from build123d import *

# Parameters (mm, degrees)
SKETCH1_W                 = 30
SKETCH1_H                 = 28
SKETCH1_R                 = 11
BOSS_EXTRUDE1_DEPTH       = 7
SKETCH2_W                 = 5
SKETCH2_H                 = 2.5
BOSS_EXTRUDE2_DEPTH       = 13
CHAMFER2_SIZE             = 2
BOSS_EXTRUDE6_DEPTH       = 2.5
CHAMFER3_SIZE             = 2
CHAMFER4_SIZE             = 2
BOSS_EXTRUDE4_DEPTH       = 2.5
CHAMFER6_SIZE             = 2.5
CHAMFER7_SIZE             = 7
CHAMFER7_SIZE_2           = 13.165085257
SKETCH7_R                 = 1.5
CUT_EXTRUDE2_DEPTH        = 6.4
BOSS_EXTRUDE7_START       = -2.5
SKETCH8_W                 = 30
SKETCH8_H                 = 5
BOSS_EXTRUDE7_DEPTH       = 4.5
CHAMFER8_SIZE             = 4.000836323
CHAMFER8_SIZE_2           = 2.5
CUT_EXTRUDE3_START        = -3
SKETCH9_R                 = 1.5
CUT_EXTRUDE3_DEPTH        = 3
SKETCH10_W                = 5.5
SKETCH10_H                = 3
CUT_EXTRUDE4_DEPTH        = 5.6
CUT_EXTRUDE5_START        = -30
SKETCH10_2_W              = 5.5
SKETCH10_2_H              = 3
CUT_EXTRUDE5_DEPTH        = 5.6
F_1_0MM_DOWEL_HOLE1_D     = 3
F_1_0MM_DOWEL_HOLE1_DEPTH = 7.098709071
F_1_0MM_DOWEL_HOLE1_TIP   = 0.901290929


with BuildPart() as part:
    # Sketch1 → Boss-Extrude1 (new body)
    with BuildSketch(Plane.XY):
        Rectangle(SKETCH1_W, SKETCH1_H)
        Circle(SKETCH1_R, mode=Mode.SUBTRACT)
    extrude(amount=BOSS_EXTRUDE1_DEPTH)

    # Sketch2 → Boss-Extrude2 (add)
    with BuildSketch(Plane(origin=(0, 0, 0), x_dir=(-1, 0, 0), z_dir=(0, 0, -1))):
        with Locations((-12.5, -12.75)):
            Rectangle(SKETCH2_W, SKETCH2_H)
        with Locations((12.5, -12.75)):
            Rectangle(SKETCH2_W, SKETCH2_H)
    extrude(amount=BOSS_EXTRUDE2_DEPTH)

    # Chamfer2
    chamfer2_edges = [part.edges().sort_by_distance(p)[0] for p in [
        (-10, -12.75, 0),
        (10, -12.75, 0),
    ]]
    chamfer(chamfer2_edges, length=CHAMFER2_SIZE)

    # Sketch5 → Boss-Extrude6 (add)
    with BuildSketch(Plane.XZ.offset(14)):
        Polygon((-10, -2), (-10, -7.5), (10, -7.5), (10, -2), (8, 0), (-8, 0), align=None)
    extrude(amount=-BOSS_EXTRUDE6_DEPTH)

    # Chamfer3
    chamfer3_edges = [part.edges().sort_by_distance(p)[0] for p in [
        (15, 0, 7),
    ]]
    chamfer(chamfer3_edges, length=CHAMFER3_SIZE)

    # Chamfer4
    chamfer4_edges = [part.edges().sort_by_distance(p)[0] for p in [
        (-15, 0, 7),
    ]]
    chamfer(chamfer4_edges, length=CHAMFER4_SIZE)

    # Sketch4 → Boss-Extrude4 (add)
    with BuildSketch(Plane(origin=(0, 0, 0), x_dir=(-1, 0, 0), z_dir=(0, 0, -1))):
        Polygon((-15, 0), (15, 11.5), (15, 14), (-15, 14), align=None)
    extrude(amount=BOSS_EXTRUDE4_DEPTH)

    # Chamfer6
    # the kernel refuses this chamfer: 2.5 mm, written as the material it adds along each edge
    with BuildSketch(Plane(origin=(21.003247512, -2.30124488, 0), x_dir=(-0.3578006820796162, -0.9333930836859554, 0.02749587661058638), z_dir=(-0.9337461173020497, 0.35793601163245237, 0))) as chamfer6_piece_1_section:
        Polygon((CHAMFER6_SIZE * 0.999621916911, -CHAMFER6_SIZE * 0.0274958766106), (-CHAMFER6_SIZE * 0.0274958766106, -CHAMFER6_SIZE * 0.999621916911), (0, 0), align=None)
    chamfer6_piece_1 = extrude(amount=17.263908412, mode=Mode.PRIVATE)
    chamfer6_piece_1 = chamfer6_piece_1 - Plane(origin=(0, 0, -0.835393566), x_dir=(1, 0, 0), z_dir=(0, 0, -1)) * Cylinder(11, 45, mode=Mode.PRIVATE)
    chamfer6_piece_1 = split(chamfer6_piece_1, bisect_by=Plane(origin=(15, -0.113968884, -0.835393566), z_dir=(-1, 0, 0)), keep=Keep.TOP, mode=Mode.PRIVATE)
    add(chamfer6_piece_1)
    with BuildSketch(Plane(origin=(-1.03959441, 6.148511191, 0), x_dir=(-0.35780068207961624, -0.9333930836859554, 0.02749587661058638), z_dir=(-0.9337461173020497, 0.35793601163245237, 0))) as chamfer6_piece_2_section:
        Polygon((CHAMFER6_SIZE * 0.999621916911, -CHAMFER6_SIZE * 0.0274958766106), (-CHAMFER6_SIZE * 0.0274958766106, -CHAMFER6_SIZE * 0.999621916911), (0, 0), align=None)
    chamfer6_piece_2 = extrude(amount=21.380172546, mode=Mode.PRIVATE)
    chamfer6_piece_2 = chamfer6_piece_2 - Plane(origin=(0, 0, -0.851534645), x_dir=(1, 0, 0), z_dir=(0, 0, -1)) * Cylinder(11, 53, mode=Mode.PRIVATE)
    chamfer6_piece_2 = split(chamfer6_piece_2, bisect_by=Plane(origin=(-15, 9.244820467, -0.851534645), z_dir=(1, 0, 0)), keep=Keep.TOP, mode=Mode.PRIVATE)
    add(chamfer6_piece_2)

    # Chamfer7
    # the kernel refuses this chamfer: 13.165085257, 7 mm, written as the material it adds along each edge
    with BuildSketch(Plane(origin=(-15, -11.5, 0), x_dir=(0, 0.9979482451756082, 0.06402577567608186), z_dir=(1, 0, 0))) as chamfer7_piece_1_section:
        Polygon((CHAMFER7_SIZE * 0.997948245176, -CHAMFER7_SIZE * 0.0640257756761), (-CHAMFER7_SIZE_2 * 0.0640257756781, -CHAMFER7_SIZE_2 * 0.997948245208), (0, 0), align=None)
    chamfer7_piece_1 = extrude(amount=30, mode=Mode.PRIVATE)
    chamfer7_piece_1 = chamfer7_piece_1 - Plane(origin=(0, 0, -3.073682767), x_dir=(1, 0, 0), z_dir=(0, 0, -1)) * Cylinder(11, 113, mode=Mode.PRIVATE)
    chamfer7_piece_1 = split(chamfer7_piece_1, bisect_by=Plane(origin=(-10, -8.887755394, -3.073682767), z_dir=(-1, 0, 0)), keep=Keep.TOP, mode=Mode.PRIVATE)
    chamfer7_piece_1 = split(chamfer7_piece_1, bisect_by=Plane(origin=(-12.500128058, -8.887755394, -7.5), z_dir=(0, 0, 1)), keep=Keep.TOP, mode=Mode.PRIVATE)
    add(chamfer7_piece_1)
    with BuildSketch(Plane(origin=(-15, -11.5, 0), x_dir=(0, 0.9979482451756082, 0.06402577567608186), z_dir=(1, 0, 0))) as chamfer7_piece_2_section:
        Polygon((CHAMFER7_SIZE * 0.997948245176, -CHAMFER7_SIZE * 0.0640257756761), (-CHAMFER7_SIZE_2 * 0.0640257756781, -CHAMFER7_SIZE_2 * 0.997948245208), (0, 0), align=None)
    chamfer7_piece_2 = extrude(amount=30, mode=Mode.PRIVATE)
    chamfer7_piece_2 = split(chamfer7_piece_2, bisect_by=Plane(origin=(-10, -10.721530873, -9.597564575), z_dir=(-1, 0, 0)), keep=Keep.TOP, mode=Mode.PRIVATE)
    chamfer7_piece_2 = split(chamfer7_piece_2, bisect_by=Plane(origin=(-12.5, -10.721530873, -7.5), z_dir=(0, 0, -1)), keep=Keep.TOP, mode=Mode.PRIVATE)
    chamfer7_piece_2 = split(chamfer7_piece_2, bisect_by=Plane(origin=(-12.5, -10.721530873, -13), z_dir=(0, 0, 1)), keep=Keep.TOP, mode=Mode.PRIVATE)
    add(chamfer7_piece_2)
    with BuildSketch(Plane(origin=(-15, -11.5, 0), x_dir=(0, 0.9979482451756082, 0.06402577567608186), z_dir=(1, 0, 0))) as chamfer7_piece_3_section:
        Polygon((CHAMFER7_SIZE * 0.997948245176, -CHAMFER7_SIZE * 0.0640257756761), (-CHAMFER7_SIZE_2 * 0.0640257756781, -CHAMFER7_SIZE_2 * 0.997948245208), (0, 0), align=None)
    chamfer7_piece_3 = extrude(amount=30, mode=Mode.PRIVATE)
    chamfer7_piece_3 = chamfer7_piece_3 - Plane(origin=(0, 0, -3.793876077), x_dir=(1, 0, 0), z_dir=(0, 0, -1)) * Cylinder(11, 113, mode=Mode.PRIVATE)
    chamfer7_piece_3 = split(chamfer7_piece_3, bisect_by=Plane(origin=(-10, -6.598719884, -3.793876077), z_dir=(1, 0, 0)), keep=Keep.TOP, mode=Mode.PRIVATE)
    chamfer7_piece_3 = split(chamfer7_piece_3, bisect_by=Plane(origin=(-9.499486782, -6.598719884, -7.5), z_dir=(0, 0, 1)), keep=Keep.TOP, mode=Mode.PRIVATE)
    chamfer7_piece_3 = split(chamfer7_piece_3, bisect_by=Plane(origin=(10, -6.598719884, -3.793876077), z_dir=(-1, 0, 0)), keep=Keep.TOP, mode=Mode.PRIVATE)
    add(chamfer7_piece_3)
    with BuildSketch(Plane(origin=(-15, -11.5, 0), x_dir=(0, 0.9979482451756082, 0.06402577567608186), z_dir=(1, 0, 0))) as chamfer7_piece_4_section:
        Polygon((CHAMFER7_SIZE * 0.997948245176, -CHAMFER7_SIZE * 0.0640257756761), (-CHAMFER7_SIZE_2 * 0.0640257756781, -CHAMFER7_SIZE_2 * 0.997948245208), (0, 0), align=None)
    chamfer7_piece_4 = extrude(amount=30, mode=Mode.PRIVATE)
    chamfer7_piece_4 = split(chamfer7_piece_4, bisect_by=Plane(origin=(12.5, -10.721530873, -7.5), z_dir=(0, 0, -1)), keep=Keep.TOP, mode=Mode.PRIVATE)
    chamfer7_piece_4 = split(chamfer7_piece_4, bisect_by=Plane(origin=(10, -10.721530873, -9.597564575), z_dir=(1, 0, 0)), keep=Keep.TOP, mode=Mode.PRIVATE)
    chamfer7_piece_4 = split(chamfer7_piece_4, bisect_by=Plane(origin=(12.5, -10.721530873, -13), z_dir=(0, 0, 1)), keep=Keep.TOP, mode=Mode.PRIVATE)
    add(chamfer7_piece_4)
    with BuildSketch(Plane(origin=(-15, -11.5, 0), x_dir=(0, 0.9979482451756082, 0.06402577567608186), z_dir=(1, 0, 0))) as chamfer7_piece_5_section:
        Polygon((CHAMFER7_SIZE * 0.997948245176, -CHAMFER7_SIZE * 0.0640257756761), (-CHAMFER7_SIZE_2 * 0.0640257756781, -CHAMFER7_SIZE_2 * 0.997948245208), (0, 0), align=None)
    chamfer7_piece_5 = extrude(amount=30, mode=Mode.PRIVATE)
    chamfer7_piece_5 = chamfer7_piece_5 - Plane(origin=(0, 0, -3.073682766), x_dir=(1, 0, 0), z_dir=(0, 0, -1)) * Cylinder(11, 113, mode=Mode.PRIVATE)
    chamfer7_piece_5 = split(chamfer7_piece_5, bisect_by=Plane(origin=(12.500128057, -8.887755394, -7.5), z_dir=(0, 0, 1)), keep=Keep.TOP, mode=Mode.PRIVATE)
    chamfer7_piece_5 = split(chamfer7_piece_5, bisect_by=Plane(origin=(10, -8.887755394, -3.073682766), z_dir=(1, 0, 0)), keep=Keep.TOP, mode=Mode.PRIVATE)
    add(chamfer7_piece_5)

    # Sketch7 → Cut-Extrude2 (cut)
    with BuildSketch(Plane.XZ.offset(14)):
        with Locations(Location((-11, 2.5, 0), (0, 0, 270))):
            Circle(SKETCH7_R)
        with Locations(Location((11, 2.5, 0), (0, 0, 270))):
            Circle(SKETCH7_R)
    extrude(amount=-CUT_EXTRUDE2_DEPTH, mode=Mode.SUBTRACT)

    # Sketch8 → Boss-Extrude7 (add)
    with BuildSketch(Plane(origin=(0, 14, 0), x_dir=(1, 0, 0), z_dir=(0, 1, 0)).offset(BOSS_EXTRUDE7_START)):
        with Locations((0, 5)):
            Rectangle(SKETCH8_W, SKETCH8_H)
    extrude(amount=BOSS_EXTRUDE7_DEPTH)

    # Chamfer8
    # the kernel refuses this chamfer: 4.000836323, 2.5 mm, written as the material it adds along each edge
    with BuildSketch(Plane(origin=(-25.343554005, 11.5, -2.5), x_dir=(0, -0.9997899140358645, 0.02049701910421793), z_dir=(1, 0, 0))) as chamfer8_piece_1_section:
        Polygon((CHAMFER8_SIZE * 0.999789913937, CHAMFER8_SIZE * 0.0204970191022), (-CHAMFER8_SIZE_2 * 0.0204970191042, CHAMFER8_SIZE_2 * 0.999789914036), (0, 0), align=None)
    chamfer8_piece_1 = extrude(amount=40.343554005, mode=Mode.PRIVATE)
    chamfer8_piece_1 = split(chamfer8_piece_1, bisect_by=Plane(origin=(2.975759377, 8.202968449, -5.855581208), z_dir=(0.25309898105600476, 0.6602582114512465, 0.707106781186274)), keep=Keep.TOP, mode=Mode.PRIVATE)
    add(chamfer8_piece_1)

    # Sketch9 → Cut-Extrude3 (cut)
    # profile 1 of 2: a face of its own
    with BuildSketch(Plane.XZ.offset(14).offset(CUT_EXTRUDE3_START)):
        Polygon((7.824573519, 2.5), (9.41228676, -0.25), (12.58771324, -0.25), (14.175426481, 2.5), (12.58771324, 5.25), (9.41228676, 5.25), align=None)
        with Locations(Location((11, 2.5, 0), (0, 0, 270))):
            Circle(SKETCH9_R, mode=Mode.SUBTRACT)
    # profile 2 of 2: a face of its own
    with BuildSketch(Plane.XZ.offset(14).offset(CUT_EXTRUDE3_START)):
        Polygon((-7.824573519, 2.5), (-9.41228676, 5.25), (-12.58771324, 5.25), (-14.175426481, 2.5), (-12.58771324, -0.25), (-9.41228676, -0.25), align=None)
        with Locations(Location((-11, 2.5, 0), (0, 0, 270))):
            Circle(SKETCH9_R, mode=Mode.SUBTRACT)
    extrude(amount=-CUT_EXTRUDE3_DEPTH, mode=Mode.SUBTRACT)

    # Sketch10 → Cut-Extrude4 (cut)
    with BuildSketch(Plane(origin=(15, 0, 0), x_dir=(0, 0, -1), z_dir=(1, 0, 0))):
        with Locations((-2.5, -9.5)):
            Rectangle(SKETCH10_W, SKETCH10_H)
    extrude(amount=-CUT_EXTRUDE4_DEPTH, mode=Mode.SUBTRACT)

    # Sketch10<2> → Cut-Extrude5 (cut)
    with BuildSketch(Plane(origin=(15, 0, 0), x_dir=(0, 0, -1), z_dir=(1, 0, 0)).offset(CUT_EXTRUDE5_START)):
        with Locations((-2.5, -9.5)):
            Rectangle(SKETCH10_2_W, SKETCH10_2_H)
    extrude(amount=CUT_EXTRUDE5_DEPTH, mode=Mode.SUBTRACT)

    # Ø1.0mm Dowel Hole1
    with Locations(Plane(origin=(0, 14, 0), x_dir=(1, 0, 0), z_dir=(0, 1, 0))):
        with Locations((-11.6, -1.25), (11.6, -1.25)):
            Hole(F_1_0MM_DOWEL_HOLE1_D / 2, depth=F_1_0MM_DOWEL_HOLE1_DEPTH)
            with Locations((0, 0, -(F_1_0MM_DOWEL_HOLE1_DEPTH + F_1_0MM_DOWEL_HOLE1_TIP / 2))):  # 118° drill point
                Cone(0, F_1_0MM_DOWEL_HOLE1_D / 2, F_1_0MM_DOWEL_HOLE1_TIP, mode=Mode.SUBTRACT)


solid = part.part
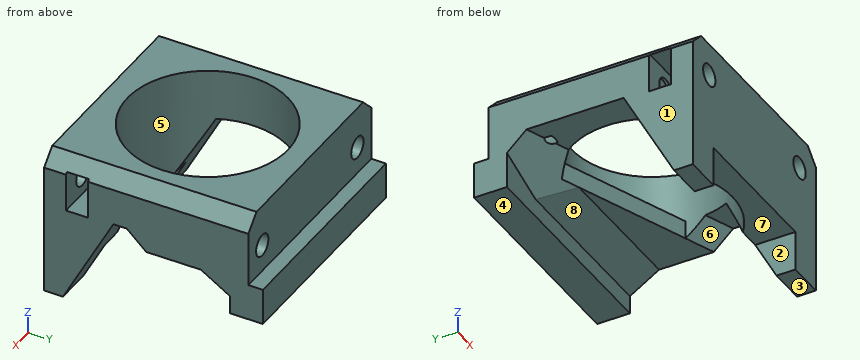
Read the model definition and answer for the solid it produces. Units are mm, in the model's axes. Face numbers are marked on the shaded views. A direction names the side the tool comes from. Give positions to 0.01 mm unless a question says otherwise; leave off trailing zeros. Loops run counter-clockwise (first coordinate to the right, second up) from the corner with the lowest first, then second, coordinate; pieces in that order, holes last. Notation, with made-up numbers: (8, 67.25) -> (46, 67.25) arc R9 cw to (46, 84.25) -> close; hole circle Ø9 at (43.25, 5). An arc over 180 degrees is marked (long way). Use a Markdown table: item, result.
Q1. Section B-B, the plane y = 12.5 is taken. Determine the outline of the cut face in (x, z), then the cut area to 3 significant figures.
Solved:
| item | result |
|---|---|
| outline | (-15, -7.5) -> (15, -7.5) -> (15, 5) -> (13, 7) -> (-13, 7) -> (-15, 5) -> close; hole circle Ø3 at (-11.6, 1.25); hole circle Ø3 at (11.6, 1.25) |
| area | 417 mm^2 |
Q2. Find the intervals of material crossed by line 1 along X through (y, z) = (-12.7, 2.5); line 2 along X through (y, z) = (-7.7, 2.5); line 3 along X through (y, z) = (-6.25, 2.5), in increasing order.
Solved:
| item | result |
|---|---|
| line 1 | x = -15 to -12.5, -9.5 to 9.5, 12.5 to 15 |
| line 2 | x = -15 to -12.5, -9.5 to -7.86, 7.86 to 9.5, 12.5 to 15 |
| line 3 | x = -15 to -9.05, 9.05 to 15 |
Q3. Section A-A, the plane x = 0.5 is taken. Determine the outline of the cut face in (y, z).
Solved:
| item | result |
|---|---|
| outline | (-14, -7.5) -> (-10.99, -7.5) -> (-10.99, 7) -> (-14, 7) -> close; (5.56, -2.5) -> (7.5, -2.5) -> (11.5, -5) -> (11.5, -7.5) -> (16, -7.5) -> (16, -2.5) -> (14, -2.5) -> (14, 7) -> (10.99, 7) -> (10.99, 0) -> (5.56, 0) -> close |
Q4. Section D-D, the plane z = -9.75 is taken. Determine the outline of the cut face in (x, y), then the cut area to 3 significant figures.
Solved:
| item | result |
|---|---|
| outline | (-15, -14) -> (-10, -14) -> (-10, -9.68) -> (-15, -9.68) -> close; (10, -14) -> (15, -14) -> (15, -9.68) -> (10, -9.68) -> close |
| area | 43.2 mm^2 |
Q5. Determine the mould class of the marked faces 1, 2 and 3 for opening direction X: pulls with the +X half, pulls with the -X half, needs draft (parallel to the pull), parting line crosses it, or undercut.
Solved:
| item | result |
|---|---|
| face 1 | pulls with the -X half |
| face 2 | undercut |
| face 3 | needs draft |
Q6. Each of these flat-tipped pins is pushed along its axis until it touches: pin 1 (12 mm diameter, centred on x = 8, z = -10, fed in from +Y); pin 2 (3.5 mm diameter, centred on x = -11.6, z = 1.25, fed in from +Y); pin 3 (1.7 mm diameter, centred on x = -2.5, y = -12.5, fed in from -Z); pin 4 (3 mm diameter, centred on x = 5, y = 4, fed in from +Z). Where does it stop, or does it pass through?
Solved:
| item | result |
|---|---|
| pin 1 | stops at y = 16 |
| pin 2 | stops at y = 14 |
| pin 3 | stops at z = -7.5 |
| pin 4 | stops at z = 0 |
Q7. A tool of negligible diameter and unlimited length cuts with its end or side. For the marked faces 4, 5, 6, 7 and 8, from which of +Z, -Z, +X, -X, +Y, -Y can it reach the whole face along a straight path? Write none if from no direction.
Solved:
| item | result |
|---|---|
| face 4 | -Z, +X, -X, +Y |
| face 5 | +Z |
| face 6 | -Z, -X |
| face 7 | -Z, +Y, -Y |
| face 8 | -Z, +X, -X |
Q8. Section C-C, the plane y = 5 is taken. Determine the outline of the cut face in (x, z), then the cut area to 3 significant figures.
Solved:
| item | result |
|---|---|
| outline | (-15, 0) -> (-9.8, 0) -> (-9.8, 7) -> (-13, 7) -> (-15, 5) -> close; (1.96, -2.5) -> (15, -2.5) -> (15, 5) -> (13, 7) -> (9.8, 7) -> (9.8, 0) -> (1.96, 0) -> close |
| area | 101 mm^2 |
